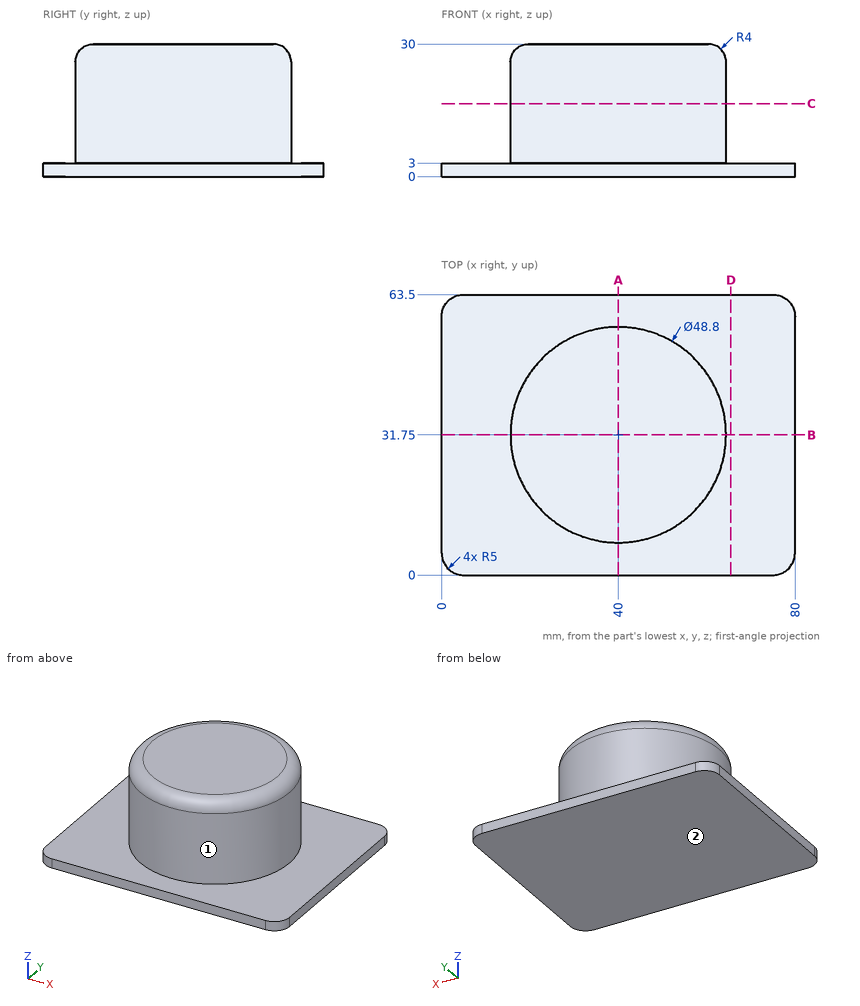
Design review of the part shown in the three views and the two pictorial views. Dimensions are in mm from the part's minimum x, y and z. A direction names the side the tool comes from. Coordinates: 2 decimals unless noted, no trailing zeros. Loops run counter-clockwise (first coordinate to the right, second up) from the corner with the lowest first, then second, coordinate; pieces in that order, holes last. Notation, with made-up numbers: (31, 1.5) - (77, 1.5) arc R25 ccw to (77, 37.5) - close; hole circle Ø2 at (70, 49.25). An arc over 180 degrees is marked (long way). Use a Markdown table: item, result. Add a question column.
Item 1: We need section D-D (x = 65.5). Give the boundary of the cut face in (y, z), and give its area (4 significant figures).
Item 2: For line 1 (Y direction, x = 40.5, z = 12.25); line 2 (Y direction, x = 50, z = 29.25); line 3 (Z direction, x = 15.5, y = 37.5), list the stretches that pass through material, from the lowest coordinate up.
Item 3: We need section A-A (x = 40). Give the boundary of the cut face in (y, z), and give its area (3 significant figures).
Item 4: We need section B-B (y = 31.75). Give the boundary of the cut face in (x, z), and give its area (3 significant figures).
Item 5: Tool access review of the marked faces 1 and 2: name each direction out of +Z, -Z, +X, -X, +Y, -Y from which nothing blocks a thin tool from reaching the whole face with its end or side.
Item 6: Insertion check: pin 1 Ø10 at (x, z) = (45, 16.5) entering from -Y; pin 2 Ø1.5 at (y, z) = (48, 22.5) entering from +X; pin 3 Ø1 at (x, z) = (63, 6.5) entering from +Y; pin 4 Ø6 at (x, z) = (10.5, 12) entering from +Y. Each pin has a flat end and moves straight along its axis. Give the tip position at first contact, or say it passes through.
Item 7: We need section C-C (z = 16.5). Give the boundary of the cut face in (x, y), and give its area (3 significant figures).
Results list:
| question | item | result |
|---|---|---|
| 1 | outline | (0, 0) - (63.5, 0) - (63.5, 3) - (0, 3) - close |
| 1 | area | 190.5 mm^2 |
| 2 | line 1 | y = 7.36 to 56.14 |
| 2 | line 2 | y = 11.34 to 52.16 |
| 2 | line 3 | z = 0 to 3 |
| 3 | outline | (0, 0) - (63.5, 0) - (63.5, 3) - (56.15, 3) - (56.15, 26) arc R4 ccw to (52.15, 30) - (11.35, 30) arc R4 ccw to (7.35, 26) - (7.35, 3) - (0, 3) - close |
| 3 | area | 1,500 mm^2 |
| 4 | outline | (0, 0) - (80, 0) - (80, 3) - (64.4, 3) - (64.4, 26) arc R4 ccw to (60.4, 30) - (19.6, 30) arc R4 ccw to (15.6, 26) - (15.6, 3) - (0, 3) - close |
| 4 | area | 1,550 mm^2 |
| 5 | face 1 | +Z |
| 5 | face 2 | -Z, +X, -X, +Y, -Y |
| 6 | pin 1 | stops at y = 7.35 |
| 6 | pin 2 | stops at x = 58.84 |
| 6 | pin 3 | stops at y = 41.19 |
| 6 | pin 4 | passes through |
| 7 | outline | circle Ø48.8 at (40, 31.75) |
| 7 | area | 1,870 mm^2 |
